```python
from build123d import *

# Parameters (mm, degrees)
SKETCH_W     = 20
SKETCH_H     = 18
PAD_DEPTH    = 5
SKETCH001_R  = 1.9
PAD001_DEPTH = 4.5
SKETCH002_R  = 1.7
HOLE_DEPTH   = 62.0711322935
POCKET_DEPTH = 2.15
CHAMFER_SIZE = 0.5
FILLET001_R  = 2


with BuildPart() as part:
    # Sketch → Pad (new body)
    with BuildSketch(Plane.YZ):
        with Locations((0, 9)):
            Rectangle(SKETCH_W, SKETCH_H)
    extrude(amount=-PAD_DEPTH)

    # Sketch001 (on Face6 of Pad) → Pad001 (join)
    with BuildSketch(Plane(origin=(-5, 0, 0), x_dir=(0, 1, 0), z_dir=(-1, 0, 0))):
        with Locations((0, -4)):
            Circle(SKETCH001_R)
    extrude(amount=PAD001_DEPTH)

    # Sketch002 (on Face5 of Pad001) → Hole (cut, through all)
    with BuildSketch(Plane(origin=(-5, 0, 0), x_dir=(0, 1, 0), z_dir=(-1, 0, 0))):
        with Locations((5.5, -12)):
            Circle(SKETCH002_R)
    hole = extrude(amount=-HOLE_DEPTH, mode=Mode.SUBTRACT)

    # Sketch003 (on Face4 of Hole) → Pocket (cut)
    with BuildSketch(Plane.YZ):
        Polygon((2.1513684387, 12), (3.8256842194, 9.1), (7.1743157806, 9.1), (8.8486315613, 12), (7.1743157806, 14.9), (3.8256842194, 14.9), align=None)
    pocket = extrude(amount=-POCKET_DEPTH, mode=Mode.SUBTRACT)

    # Mirrored: Hole, Pocket across XZ
    add(hole.mirror(Plane.XZ), mode=Mode.SUBTRACT)
    add(pocket.mirror(Plane.XZ), mode=Mode.SUBTRACT)

    # Chamfer
    chamfer_edges = [part.edges().sort_by_distance(p)[0] for p in [
        (-9.5, -1.9, 4),
    ]]
    chamfer(chamfer_edges, length=CHAMFER_SIZE)

    # Fillet001
    fillet001_edges = [part.edges().sort_by_distance(p)[0] for p in [
        (-2.5, 10, 0),
        (-2.5, -10, 0),
    ]]
    fillet(fillet001_edges, radius=FILLET001_R)


solid = part.part
```
For this review, take the finished solid that the model builds, in its own axes (mm). A direction names the side the tool comes from. Give positions to 0.01 mm unless a question says otherwise; leave off trailing zeros. Order: outer loops, then holes, each group sorted by start corner. A loop starts at its lowest first (then second) coordinate and runs counter-clockwise, first axis right, second up.
1) Take a section at D-D (x = -8). Give the boundary of the cut face in (y, z).
2) Take a section at B-B (x = -1.25). Give the boundary of the cut face in (y, z).
3) For faces 1 (the face through (-1, -6, 14.9)), 2 (the face through (-9.5, 0, 4)), list the 3-axis set-ups (+Z, -Z, +X, -X, +Y, -Y) from which the entire face can be reached by the end or side of a thin tool; tool diameter is ignored.
4) Take a section at A-A (y = 5.5). Give the boundary of the cut face in (x, z), then the cut area to 3 significant figures.
5) The part is to be moulded in two halves that separate along Z. For faces 3 (the face through (-1.06, -8, 10.53)), 4 (the face through (-6.972, -0.247, 2.116)), 5 (the face through (-2, -10, 10)), say which applies: released by +Z, released by -Z, zero draft, split by the parting line, or undercut.
6) Wall thickness on line 1 (Y direction, x = -3.3, z = 12); line 2 (Z direction, x = -3.7, y = 5.5); line 3 (X direction, y = 7, z = 4.25): over which ranges is each line inside the solid? List them lowest first.
7) Take a section at C-C (z = 4). Give the boundary of the cut face in (x, y).
8) Insertion check: pin 1 (8 mm diameter, centred on y = 1.5, z = 5, fed in from +X); pin 2 (4 mm diameter, centred on y = 5.5, z = 12, fed in from -X); pin 3 (3 mm diameter, centred on y = -5.5, z = 11.5, fed in from +X); pin 4 (4 mm diameter, centred on y = -1.5, z = 7.5, fed in from -X). Each pin has a flat end and moves straight along its axis. Give the tip position at first contact, or say it passes through.
Derived:
1. outline: circle Ø3.8 at (0, 4)
2. outline: (-10, 2) arc R2 ccw to (-8, 0) - (8, 0) arc R2 ccw to (10, 2) - (10, 18) - (-10, 18) - close; hole (-8.85, 12) - (-7.17, 9.1) - (-3.83, 9.1) - (-2.15, 12) - (-3.83, 14.9) - (-7.17, 14.9) - close; hole (2.15, 12) - (3.83, 9.1) - (7.17, 9.1) - (8.85, 12) - (7.17, 14.9) - (3.83, 14.9) - close
3. face 1: +X
3. face 2: +Z, -Z, -X, +Y, -Y
4. outline: (-5, 0) - (0, 0) - (0, 9.1) - (-2.15, 9.1) - (-2.15, 10.3) - (-5, 10.3) - close; (-5, 13.7) - (-2.15, 13.7) - (-2.15, 14.9) - (0, 14.9) - (0, 18) - (-5, 18) - close
4. area: 67.8 mm2
5. face 3: undercut
5. face 4: split by the parting line
5. face 5: zero draft
6. line 1: y = -10 to -7.2, -3.8 to 3.8, 7.2 to 10
6. line 2: z = 0 to 10.3, 13.7 to 18
6. line 3: x = -5 to 0
7. outline: (-9.5, -1.4) - (-9, -1.9) - (-5, -1.9) - (-5, -10) - (0, -10) - (0, 10) - (-5, 10) - (-5, 1.9) - (-9, 1.9) - (-9.5, 1.4) - close
8. pin 1: stops at x = 0
8. pin 2: stops at x = -5
8. pin 3: stops at x = -2.15
8. pin 4: stops at x = -9.09
